```python
from build123d import *

# Parameters (mm, degrees)
F0_R     = 8.5
F1_DEPTH = 4
F2_R     = 5
F3_DEPTH = 100


with BuildPart() as f1:
    # F0 (on Top) → F1 (new body)
    with BuildSketch(Plane.XY):
        Circle(F0_R)
    extrude(amount=F1_DEPTH)

    # F2 (on Top) → F3 (join)
    with BuildSketch(Plane.XY):
        Circle(F2_R)
    extrude(amount=F3_DEPTH)

    # F4 (on Right) → F5 (revolve)
    with BuildSketch(Plane.YZ):
        with BuildLine():
            Line((0, 102), (0, 100))
            Line((0, 100), (5, 100))
            ThreePointArc((5, 100), (3.585786, 100.585786), (3, 102))
            Line((3, 102), (0, 102))
        make_face()
    revolve(axis=Axis((0, 0, 101), (0, 0, 1)))


solid = f1.part
```
Input: part model. Units: mm. Frame: model coordinates. A direction names the side the tool comes from. Round coordinates to 2 decimals unless told otherwise and drop trailing zeros. Loops run counter-clockwise (first coordinate to the right, second up) from the corner with the lowest first, then second, coordinate; pieces in that order, holes last.
1) Pin query (flat end, axial travel): pin 1 (3 mm diameter, centred on y = -1.5, z = 74, fed in from -X); pin 2 (6 mm diameter, centred on x = 5.5, z = 26, fed in from -Y); pin 3 (3 mm diameter, centred on y = 5, z = 35.5, fed in from +X). Return the tip coordinate at first contact, or that it passes through.
Ans:
pin 1: stops at x = -5
pin 2: stops at y = -4.33
pin 3: stops at x = 3.57
2) Section query D-D on y = 7.5. Return the cut outline in (x, z), plus the area to 3 significant figures.
Ans:
outline: (-4, 0) - (4, 0) - (4, 4) - (-4, 4) - close
area: 32.0 mm2
3) Section query C-C on z = 80. Return the cut outline in (x, y), plus the area to 3 significant figures.
Ans:
outline: circle Ø10 at (0, 0)
area: 78.5 mm2
4) Set-up query: faces 1 (the cylindrical face through (4.57, 7.167, 1.972)), 2 (the flat face through (4, -4, 4)). Return all of +Z, -Z, +X, -X, +Y, -Y with unobstructed straight access to the full face (end or side cutting, diameter ignored); none if empty.
Ans:
face 1: +Z, -Z
face 2: +Z
5) Material intervals for line 1 (Z direction, x = 3.25, y = -5.5); line 2 (X direction, y = 0.25, z = 97.5); line 3 (X direction, y = -4, z = 25.5), sorted ascending.
Ans:
line 1: z = 0 to 4
line 2: x = -4.99 to 4.99
line 3: x = -3 to 3
6) Section query A-A on y = 0. Return the cut outline in (x, z), plus the area to 3 significant figures.
Ans:
outline: (-8.5, 0) - (8.5, 0) - (8.5, 4) - (5, 4) - (5, 100) arc R2 cw to (3, 102) - (-3, 102) arc R2 cw to (-5, 100) - (-5, 4) - (-8.5, 4) - close
area: 1,040 mm2
